```python
from build123d import *

# Parameters (mm, degrees)
EXTRUDE_1_DEPTH = 570


with BuildPart() as part:
    # 草图1 → 凸台-拉伸1 (new body)
    with BuildSketch(Plane.XY):
        with BuildLine():
            Line((-12.404964531, 1), (325.76800896, 1))
            ThreePointArc((325.76800896, 1), (345.710427238, -41.682324575), (300.176786305, -29.59231129))
            ThreePointArc((300.176786305, -29.59231129), (294.936443949, -20.563156945), (285.123660003, -17))
            Line((285.123660003, -17), (-12.404964531, -17))
            ThreePointArc((-12.404964531, -17), (-21.404964531, -8), (-12.404964531, 1))
        make_face()
        with BuildLine():
            Line((-12.404964531, 0), (325.76800896, 0))
            ThreePointArc((325.76800896, 0), (344.943411151, -41.040696707), (301.161064099, -29.415683933))
            ThreePointArc((301.161064099, -29.415683933), (295.578071817, -19.796140858), (285.123660003, -16))
            Line((285.123660003, -16), (-12.404964531, -16))
            ThreePointArc((-12.404964531, -16), (-20.404964531, -8), (-12.404964531, 0))
        make_face(mode=Mode.SUBTRACT)
    extrude(amount=EXTRUDE_1_DEPTH)


solid = part.part
```
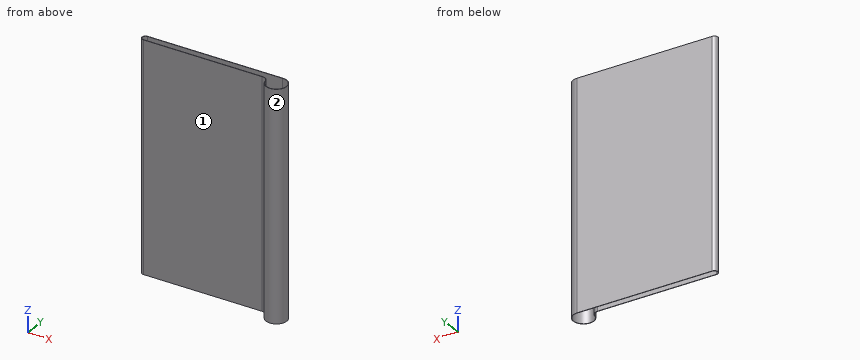
Part model, mm, in its own coordinate system. Face numbers are marked on the shaded views. A direction names the side the tool comes from. Give positions to 0.01 mm unless a question says otherwise; leave off trailing zeros. Write each loop counter-clockwise with the first axis right and the second up, starting at its lowest first coordinate (ties: lowest second). Pieces come first, ordered by that corner, then holes. Notation, with made-up numbers: (51.25, 50) -> (64.25, 50) arc R17 ccw to (64.25, 65) -> close; hole circle Ø3 at (-16.5, 38.25). An arc over 180 degrees is marked (long way). Put each result on its own line as item: value. Start each with the question number.
Item 1: Cut at C-C (y = -8). List the corners of the cut face in (x, z), then the cut area to 3 significant figures.
Item 2: Cut at A-A (x = 254.5). List the corners of the cut face in (y, z), then the cut area to 3 significant figures.
Item 3: Pin check, flat tips, straight feed: pin 1 Ø6 at (y, z) = (-9.5, 297) entering from +X; pin 2 Ø10 at (x, y) = (70, -26) entering from -Z; pin 3 Ø8 at (y, z) = (-27, 291) entering from -X. Stop position of each tip, or through.
Item 4: Which spindle directions (+Z, -Z, +X, -X, +Y, -Y) get a long thin tool onto all of the face, cutting with end or side? Do the marked faces 1 and 2. Say none if no direction does.
Item 5: Cut at B-B (z = 35). List the corners of the cut face in (x, y).
Item 6: Wall check: L1, parallel to Y at x = 98.5, z = 35.5; L2, parallel to X at y = -25, z = 235; L3, parallel to X at y = -21.5, z = 217. Give the ranges that are in metal, low to high. Write a range as [from, to].
Answer list:
1. outline: (-21.4, 0) -> (-20.4, 0) -> (-20.4, 570) -> (-21.4, 570) -> close; (344.1, 0) -> (345.44, 0) -> (345.44, 570) -> (344.1, 570) -> close
1. area: 1,330 mm2
2. outline: (-17, 0) -> (-16, 0) -> (-16, 570) -> (-17, 570) -> close; (0, 0) -> (1, 0) -> (1, 570) -> (0, 570) -> close
2. area: 1,140 mm2
3. pin 1: stops at x = 348.57
3. pin 2: passes through
3. pin 3: stops at x = 297.27
4. face 1: +Z, -Z, -X, -Y
4. face 2: +Z, -Z
5. outline: (-12.4, -17) -> (285.12, -17) arc R15.29 cw to (300.18, -29.59) arc R26 ccw (long way) to (325.77, 1) -> (-12.4, 1) arc R9 ccw to start; hole (-12.4, -16) -> (285.12, -16) arc R16.29 cw to (301.16, -29.42) arc R25 ccw (long way) to (325.77, 0) -> (-12.4, 0) arc R8 ccw to start
6. L1: y = [-17, -16], [0, 1]
6. L2: x = [298.57, 299.69], [350.77, 351.77]
6. L3: x = [295.96, 297.33], [350.52, 351.53]
